The listing builds one solid part. Answer for the finished solid, in the listing's coordinates (mm). Face numbers are marked on the shaded views. A direction names the side the tool comes from. Give positions to 0.01 mm unless a question says otherwise; leave off trailing zeros. Write each loop counter-clockwise with the first axis right and the second up, starting at its lowest first coordinate (ties: lowest second). Pieces come first, ordered by that corner, then holes. Notation, with made-up numbers: (9.25, 11.5) -> (31.25, 11.5) arc R20 ccw to (31.25, 22.5) -> close; hole circle Ø10 at (31, -25.75). An arc over 180 degrees is marked (long way). One line per question, with ' | ' between items.
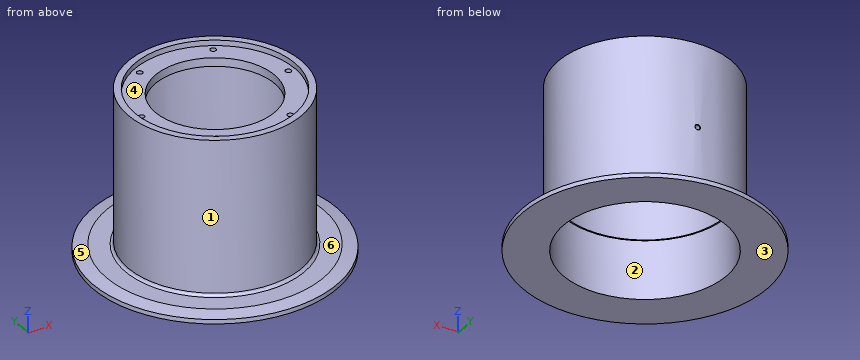
from build123d import *

# Parameters (mm, degrees)
SKETCH_1_R                    = 180
EXTRUDE_1_DEPTH               = 10
SKETCH_2_R                    = 128
EXTRUDE_2_DEPTH               = 238
SKETCH_3_R                    = 120
CUT_EXTRUDE_1_DEPTH           = 86
SKETCH_4_R                    = 118
CUT_EXTRUDE_2_DEPTH           = 131.5
SKETCH_5_R                    = 88
CUT_EXTRUDE_3_DEPTH           = 335.822714283
CUT_EXTRUDE_START             = -8
SKETCH_6_R                    = 118
CUT_EXTRUDE_4_DEPTH           = 8
HOLE_WIZARD_M10_1_D           = 8.5
HOLE_WIZARD_M10_1_CSINK_D     = 8.55
HOLE_WIZARD_M10_1_CSINK_ANGLE = 90
FILLET_1_R                    = 4
CHAMFER_1_SIZE                = 20
CHAMFER_1_SIZE2               = 3.526539614


# Read off the part's stored shape, not the designer's step: M8 螺纹孔1
with BuildPart() as part:
    # 草图1 → 凸台-拉伸1 (new body)
    with BuildSketch(Plane.XY):
        Circle(SKETCH_1_R)
    extrude(amount=EXTRUDE_1_DEPTH)

    # 草图2 → 凸台-拉伸2 (add)
    with BuildSketch(Plane.XY):
        Circle(SKETCH_2_R)
    extrude(amount=EXTRUDE_2_DEPTH)

    # 草图3 → 切除-拉伸1 (cut)
    with BuildSketch(Plane(origin=(0, 0, 0), x_dir=(-1, 0, 0), z_dir=(0, 0, -1))):
        Circle(SKETCH_3_R)
    extrude(amount=-CUT_EXTRUDE_1_DEPTH, mode=Mode.SUBTRACT)

    # 草图4 → 切除-拉伸2 (cut)
    with BuildSketch(Plane(origin=(0, 0, 86), x_dir=(-1, 0, 0), z_dir=(0, 0, -1))):
        Circle(SKETCH_4_R)
    extrude(amount=-CUT_EXTRUDE_2_DEPTH, mode=Mode.SUBTRACT)

    # 草图5 → 切除-拉伸3 (cut, through all)
    with BuildSketch(Plane(origin=(0, 0, 217.5), x_dir=(-1, 0, 0), z_dir=(0, 0, -1))):
        Circle(SKETCH_5_R)
    extrude(amount=-CUT_EXTRUDE_3_DEPTH, mode=Mode.SUBTRACT)

    # 草图6 → 切除-拉伸4 (cut)
    with BuildSketch(Plane.XY.offset(238).offset(CUT_EXTRUDE_START)):
        with Locations(Location((0, 0, 0), (0, 0, 180))):
            Circle(SKETCH_6_R)
    extrude(amount=CUT_EXTRUDE_4_DEPTH, mode=Mode.SUBTRACT)

    # M10 螺纹孔的螺纹孔钻头1 (through all)
    with Locations(Plane.XY.offset(230)):
        with Locations((108, 0), (54, -93.530743609), (-54, -93.530743609), (-108, 0), (-54, 93.530743609), (54, 93.530743609)):
            CounterSinkHole(HOLE_WIZARD_M10_1_D / 2, HOLE_WIZARD_M10_1_CSINK_D / 2, counter_sink_angle=HOLE_WIZARD_M10_1_CSINK_ANGLE)

    # 圆角1
    fillet_1_edges = [part.edges().sort_by_distance(p)[0] for p in [
        (-128, 0, 10),
    ]]
    fillet(fillet_1_edges, radius=FILLET_1_R)

    # 倒角1
    chamfer_1_edges = [part.edges().sort_by_distance(p)[0] for p in [
        (-180, 0, 10),
    ]]
    chamfer_1_side = [part.faces().sort_by_distance(p)[0] for p in [
        (-137.091168825, 0, 10),
    ]]
    chamfer(chamfer_1_edges, length=CHAMFER_1_SIZE, length2=CHAMFER_1_SIZE2, reference=chamfer_1_side[0])

    # M8 螺纹孔1 outline → M8 螺纹孔1 (revolve, cut)
    with BuildSketch(Plane.XY.offset(115.5)):
        Polygon((4.025021706, 128.000021706), (0, 128.000021706), (0, 117.951000003), (3.4, 117.951000003), (3.4, 127.375), align=None)
    revolve(axis=Axis((0, 0, 115.5), (0, 1, 0)), mode=Mode.SUBTRACT)


solid = part.part
Item 1: A tool of negligible diameter and unlimited length cuts with its end or side. For the marked faces 1, 2 and 3, from which of +Z, -Z, +X, -X, +Y, -Y can it reach the whole face along a straight path? Write none if from no direction.
Answers below:
face 1: +Z | face 2: -Z | face 3: -Z, +X, -X, +Y, -Y
Item 2: Find section A-A (z = 176). Write down the section's boundary in (x, y).
Answers below:
outline: circle Ø256 at (0, 0); hole circle Ø236 at (0, 0)
Item 3: Flat-ended cylindrical pins translate along their axes: pin 1 (6 mm diameter, centred on y = 59.5, z = 106.5, fed in from +X); pin 2 (10 mm diameter, centred on x = -115, y = 133, fed in from +Z); pin 3 (1.5 mm diameter, centred on x = 31.5, z = 147.5, fed in from -Y); pin 4 (7 mm diameter, centred on x = 108, y = 0, fed in from -Z). Find the tip coordinate at first contact, or state that the pin passes through.
Answers below:
pin 1: x = 114.86 | pin 2: z = 8.09 | pin 3: y = -124.25 | pin 4: through
Item 4: Consider line 1 (Y direction, x = -54, z = 223.5); line 2 (X direction, y = 73, z = 115); line 3 (Z direction, x = 72.5, y = 91.5). Determine where each line is inside the solid, lowest interval first. Write a range as [from, to].
Answers below:
line 1: [-116.05, -97.78], [-89.28, -69.48], [69.48, 89.28], [97.78, 116.05] | line 2: [-105.14, -92.71], [92.71, 105.14] | line 3: [217.5, 230]
Item 5: Determine the mould class of the marked faces 4, 5 and 6 for opening direction Y: pulls with the +Y half, pulls with the -Y half, needs draft (parallel to the pull), parting line crosses it, or undercut.
Answers below:
face 4: undercut | face 5: parting line crosses it | face 6: needs draft
